```python
from build123d import *

# Parameters (mm, degrees)
SKETCH_1_W          = 11
SKETCH_1_H          = 48
EXTRUDE_1_DEPTH     = 13
FILLET_1_R          = 2
SKETCH_5_R          = 1.525
CUT_EXTRUDE_1_DEPTH = 14


with BuildPart() as part:
    # 草图1 → 凸台-拉伸1 (new body)
    with BuildSketch(Plane(origin=(0, 0, 0), x_dir=(1, 0, 0), z_dir=(0, 1, 0))):
        Rectangle(SKETCH_1_W, SKETCH_1_H)
    extrude(amount=EXTRUDE_1_DEPTH)

    # 圆角1
    fillet_1_edges = [part.edges().sort_by_distance(p)[0] for p in [
        (5.5, 6.5, 24),
        (-5.5, 6.5, 24),
        (-5.5, 6.5, -24),
        (5.5, 6.5, -24),
    ]]
    fillet(fillet_1_edges, radius=FILLET_1_R)

    # 草图5 → 切除-拉伸1 (cut, through all)
    with BuildSketch(Plane(origin=(0, 13, 0), x_dir=(1, 0, 0), z_dir=(0, 1, 0))):
        Circle(SKETCH_5_R)
        with Locations((0, 15)):
            Circle(SKETCH_5_R)
        with Locations((0, -15)):
            Circle(SKETCH_5_R)
    extrude(amount=-CUT_EXTRUDE_1_DEPTH, mode=Mode.SUBTRACT)


solid = part.part
```
For this review, take the finished solid that the model builds, in its own axes (mm). Give positions to 0.01 mm unless a question says otherwise; leave off trailing zeros. Order: outer loops, then holes, each group sorted by start corner. A loop starts at its lowest first (then second) coordinate and runs counter-clockwise, first axis right, second up.
1) Insertion check: pin 1 (1.8 mm diameter, centred on x = 0, z = -15, fed in from -Y); pin 2 (1 mm diameter, centred on x = -1.5, z = -1, fed in from -Y). Each pin has a flat end and moves straight along its axis. Give the tip position at first contact, or say it passes through.
2) Take a section at C-C (z = -15). Give the boundary of the cut face in (x, y) (3 decimals), then the cut area to 3 significant figures.
3) Wall thickness on line 1 (Z direction, x = 0, y = 9.75) (3 decimals); line 2 (X direction, y = 6.25, z = 15) (3 decimals); line 3 (Z direction, x = 1, y = 9): over which ranges is each line inside the solid? List them lowest first.
4) Take a section at B-B (x = 0). Give the boundary of the cut face in (y, z) (3 decimals), then the cut area to 3 significant figures.
5) Take a section at A-A (y = 6). Give the boundary of the cut face in (x, z) (3 decimals), then the cut area to 3 significant figures.
Derived:
1. pin 1: passes through
1. pin 2: stops at y = 0
2. outline: (-5.5, 0) - (-1.525, 0) - (-1.525, 13) - (-5.5, 13) - close; (1.525, 0) - (5.5, 0) - (5.5, 13) - (1.525, 13) - close
2. area: 103 mm2
3. line 1: z = -24 to -16.525, -13.475 to -1.525, 1.525 to 13.475, 16.525 to 24
3. line 2: x = -5.5 to -1.525, 1.525 to 5.5
3. line 3: z = -24 to -16.15, -13.85 to -1.15, 1.15 to 13.85, 16.15 to 24
4. outline: (0, -24) - (13, -24) - (13, -16.525) - (0, -16.525) - close; (0, -13.475) - (13, -13.475) - (13, -1.525) - (0, -1.525) - close; (0, 1.525) - (13, 1.525) - (13, 13.475) - (0, 13.475) - close; (0, 16.525) - (13, 16.525) - (13, 24) - (0, 24) - close
4. area: 505 mm2
5. outline: (-5.5, -22) arc R2 ccw to (-3.5, -24) - (3.5, -24) arc R2 ccw to (5.5, -22) - (5.5, 22) arc R2 ccw to (3.5, 24) - (-3.5, 24) arc R2 ccw to (-5.5, 22) - close; hole circle Ø3.05 at (0, -15); hole circle Ø3.05 at (0, 0); hole circle Ø3.05 at (0, 15)
5. area: 503 mm2
